Input: part model. Units: mm. Frame: model coordinates. A direction names the side the tool comes from. Coordinates: 2 decimals unless noted, no trailing zeros. Order: outer loops, then holes, each group sorted by start corner. A loop starts at its lowest first (then second) coordinate and runs counter-clockwise, first axis right, second up. Notation, with made-up numbers: (-40, 18.25) -> (-27, 18.25) arc R16 cw to (-27, 43.25) -> close; hole circle Ø5 at (24, 55.25). An arc over 180 degrees is marked (long way). Write each question's results on one line, items separated by ' | '.
```python
from build123d import *

# Parameters (mm, degrees)
SKETCH2_R          = 16.5
SKETCH2_R_2        = 12.5
CUT_EXTRUDE1_DEPTH = 7
SKETCH3_R          = 35
SKETCH3_R_2        = 27.5
CUT_EXTRUDE2_DEPTH = 3
SKETCH4_R          = 3
CUT_EXTRUDE4_DEPTH = 25


with BuildPart() as part:
    # Sketch1 → Revolve1 (revolve)
    with BuildSketch(Plane.XY):
        Polygon((0, 30), (0, 12.5), (25, 12.5), (25, 35), (5, 35), (5, 30), align=None)
    revolve(axis=Axis((25, 0, 0), (-1, 0, 0)))

    # Mirror1: part across plane


with BuildPart() as part_1:
    add(part.part)
    add(part.part.mirror(Plane(origin=(0, 0, 0), x_dir=(0, 0, 1), z_dir=(1, 0, 0))))

    # Sketch2 → Cut-Extrude1 (cut)
    with BuildSketch(Plane(origin=(25, 0, 0), x_dir=(0, 0, -1), z_dir=(1, 0, 0))):
        with Locations(Location((0, 0, 0), (0, 0, 90))):
            Circle(SKETCH2_R)
        with Locations(Location((0, 0, 0), (0, 0, 90))):
            Circle(SKETCH2_R_2, mode=Mode.SUBTRACT)
    extrude(amount=-CUT_EXTRUDE1_DEPTH, mode=Mode.SUBTRACT)

    # Sketch3 → Cut-Extrude2 (cut)
    with BuildSketch(Plane(origin=(25, 0, 0), x_dir=(0, 0, -1), z_dir=(1, 0, 0))):
        with Locations(Location((0, 0, 0), (0, 0, 90))):
            Circle(SKETCH3_R)
        with Locations(Location((0, 0, 0), (0, 0, 90))):
            Circle(SKETCH3_R_2, mode=Mode.SUBTRACT)
    extrude(amount=-CUT_EXTRUDE2_DEPTH, mode=Mode.SUBTRACT)

    # Sketch4 → Cut-Extrude4 (cut)
    with BuildSketch(Plane(origin=(0, 35, 0), x_dir=(1, 0, 0), z_dir=(0, 1, 0))):
        with Locations((13.5, 0)):
            Circle(SKETCH4_R)
    extrude(amount=-CUT_EXTRUDE4_DEPTH, mode=Mode.SUBTRACT)


solid = part_1.part
```
(1) Mould query, pull axis X, two halves, no side actions, for faces 5 (the face through (25, -12, 12)), 6 (the face through (-5, 26, -16)), 7 (the face through (-25, 0, 15)). Classes: +X half, -X half, draft (parallel to the pull), parting line (faces both ways), or undercut.
Return value:
face 5: +X half | face 6: undercut | face 7: -X half
(2) Line query: line 1 along Z through (x, y) = (-11, -0.5); line 2 along Y through (x, z) = (-3, 0); line 3 along X through (y, z) = (-25, 18.5). Output: solid intervals per line, ascending. Write a range as from..to.
Return value:
line 1: -35..-12.49, 12.49..35 | line 2: -30..-12.5, 12.5..30 | line 3: -25..-5, 5..22
(3) Cut plane D-D, the plane y = 20. Return loops of the section in (x, z), plus the area to 3 significant figures.
Return value:
outline: (-25, -28.72) -> (-5, -28.72) -> (-5, -22.36) -> (5, -22.36) -> (5, -28.72) -> (22, -28.72) -> (22, -18.87) -> (25, -18.87) -> (25, 18.87) -> (22, 18.87) -> (22, 28.72) -> (5, 28.72) -> (5, 22.36) -> (-5, 22.36) -> (-5, 28.72) -> (-25, 28.72) -> close; hole circle Ø6 at (13.5, 0) | area: 2,660 mm2
(4) Pin query (flat end, axial travel): P1, Ø1, axis at x = -6.5, z = -7.5, coming from the +Y side; P2, Ø5, axis at x = 12.5, y = 26, coming from the -Z side; P3, Ø6, axis at x = -11.5, z = 19.5, coming from the -Y side. Return the tip coordinate at first contact, or that it passes through.
Return value:
P1: y = 34.29 | P2: z = -25.94 | P3: y = -30.87
(5) Cut plane A-A, the plane z = 0. Return loops of the section in (x, y).
Return value:
outline: (-25, -35) -> (-5, -35) -> (-5, -30) -> (5, -30) -> (5, -35) -> (22, -35) -> (22, -27.5) -> (25, -27.5) -> (25, -16.5) -> (18, -16.5) -> (18, -12.5) -> (-25, -12.5) -> close; (-25, 12.5) -> (10.5, 12.5) -> (10.5, 35) -> (5, 35) -> (5, 30) -> (-5, 30) -> (-5, 35) -> (-25, 35) -> close; (16.5, 12.5) -> (18, 12.5) -> (18, 16.5) -> (25, 16.5) -> (25, 27.5) -> (22, 27.5) -> (22, 35) -> (16.5, 35) -> close
(6) Cut plane C-C, the plane z = 31.5. Return loops of the section in (x, y).
Return value:
outline: (-25, -15.26) -> (-5, -15.26) -> (-5, 15.26) -> (-25, 15.26) -> close; (5, -15.26) -> (22, -15.26) -> (22, 15.26) -> (5, 15.26) -> close
(7) Cut plane B-B, the plane y = 0. Return loops of the section in (x, z).
Return value:
outline: (-25, -35) -> (-5, -35) -> (-5, -30) -> (5, -30) -> (5, -35) -> (22, -35) -> (22, -27.5) -> (25, -27.5) -> (25, -16.5) -> (18, -16.5) -> (18, -12.5) -> (-25, -12.5) -> close; (-25, 12.5) -> (18, 12.5) -> (18, 16.5) -> (25, 16.5) -> (25, 27.5) -> (22, 27.5) -> (22, 35) -> (5, 35) -> (5, 30) -> (-5, 30) -> (-5, 35) -> (-25, 35) -> close
(8) Reachability of faces 1 (the face through (5, 26, -16)), 2 (the face through (10.5, 23.7, -0.1)), 3 (the face through (23.521, 12.69, -24.397)), 4 (the face through (-3.801, 11.923, -3.755)) from +Z, -Z, +X, -X, +Y, -Y: full face, straight path, thin tool, end or side. Return the list, or none.
Return value:
face 1: none | face 2: +Y | face 3: +X | face 4: +X, -X
